from build123d import *

# Parameters (mm, degrees)
F0_W     = 100
F0_H     = 60
F1_DEPTH = 70
F2_SIZE  = 10
F3_SIZE  = 7


with BuildPart() as f1:
    # F0 (on Top) → F1 (new body)
    with BuildSketch(Plane.XY):
        Rectangle(F0_W, F0_H)
    extrude(amount=F1_DEPTH)

    # F2
    f2_edges = [f1.edges().sort_by_distance(p)[0] for p in [
        (-50, -30, 35),
        (50, -30, 35),
        (50, 30, 35),
        (-50, 30, 35),
    ]]
    chamfer(f2_edges, length=F2_SIZE)

    # F3
    f3_edges = [f1.edges().sort_by_distance(p)[0] for p in [
        (45, 25, 70),
        (45, 25, 0),
        (-45, 25, 70),
        (-45, 25, 0),
        (-45, -25, 70),
        (45, -25, 70),
        (-45, -25, 0),
        (45, -25, 0),
    ]]
    chamfer(f3_edges, length=F3_SIZE)


solid = f1.part
Could you check a few things on this model? Use its own coordinates, in mm. Give positions to 0.01 mm unless a question says otherwise; leave off trailing zeros. Order: outer loops, then holes, each group sorted by start corner. A loop starts at its lowest first (then second) coordinate and runs counter-clockwise, first axis right, second up. Notation, with made-up numbers: (36.25, 18) - (42.25, 18) arc R24 ccw to (42.25, 55) - close; hole circle Ø9 at (-16, 0). An arc over 180 degrees is marked (long way). One line per item, written item: value. Start each with the question number.
1. Imagine slicing it at B-B on y = 26. List the corners of the cut face in (x, z) for me.
2. Imagine slicing it at A-A on z = 18. List the corners of the cut face in (x, y) for me, plus the area to 3 significant figures.
3. If I drill on probe 1 along X at (y, z) = (-27, 19.5); probe 2 along X at (y, z) = (24, 30.5), over which ranges is the centre line in solid material (lowest first)?
Values:
1. outline: (-44, 7) - (-34.1, 0) - (34.1, 0) - (44, 7) - (44, 63) - (34.1, 70) - (-34.1, 70) - (-44, 63) - close
2. outline: (-50, -20) - (-40, -30) - (40, -30) - (50, -20) - (50, 20) - (40, 30) - (-40, 30) - (-50, 20) - close
2. area: 5,800 mm²
3. probe 1: -43 to 43
3. probe 2: -46 to 46
